```python
from build123d import *

# Parameters (mm, degrees)
SKETCH1_R          = 76.2
EXTRUDE1_DEPTH     = 17.272
SKETCH2_R          = 30.099
CUT_EXTRUDE1_DEPTH = 22.352
SKETCH3_R          = 4.2164
CUT_EXTRUDE3_DEPTH = 22.352
CIRPATTERN1_COUNT  = 8
SKETCH4_R          = 4.2164
CUT_EXTRUDE4_DEPTH = 22.352
CIRPATTERN2_COUNT  = 16


with BuildPart() as part:
    # Sketch1 → Extrude1 (new body)
    with BuildSketch(Plane(origin=(0, 0, 0), x_dir=(1, 0, 0), z_dir=(0, 1, 0))):
        with Locations(Location((0, 0, 0), (0, 0, 270))):
            Circle(SKETCH1_R)
    extrude(amount=EXTRUDE1_DEPTH)

    # Sketch2 → Cut-Extrude1 (cut)
    with BuildSketch(Plane(origin=(0, 0, 0), x_dir=(1, 0, 0), z_dir=(0, 1, 0))):
        with Locations(Location((0, 0, 0), (0, 0, 270))):
            Circle(SKETCH2_R)
    extrude(amount=CUT_EXTRUDE1_DEPTH, mode=Mode.SUBTRACT)

    # Sketch3 → Cut-Extrude3 (cut)
    with BuildSketch(Plane(origin=(0, 0, 0), x_dir=(1, 0, 0), z_dir=(0, 1, 0))):
        with Locations(Location((0, 46.101, 0), (0, 0, 270))):
            Circle(SKETCH3_R)
    cut_extrude3 = extrude(amount=CUT_EXTRUDE3_DEPTH, mode=Mode.SUBTRACT)

    # CirPattern1: Cut-Extrude3 ×8 about axis
    cirpattern1_axis = Axis((0, 0, 0), (0, 1, 0))
    for i in range(1, CIRPATTERN1_COUNT):
        add(cut_extrude3.rotate(cirpattern1_axis, i * 360 / CIRPATTERN1_COUNT), mode=Mode.SUBTRACT)

    # Sketch4 → Cut-Extrude4 (cut)
    with BuildSketch(Plane(origin=(0, 0, 0), x_dir=(1, 0, 0), z_dir=(0, 1, 0))):
        with Locations(Location((0, 65.151, 0), (0, 0, 270))):
            Circle(SKETCH4_R)
    cut_extrude4 = extrude(amount=CUT_EXTRUDE4_DEPTH, mode=Mode.SUBTRACT)

    # CirPattern2: Cut-Extrude4 ×16 about axis
    cirpattern2_axis = Axis((0, 0, 0), (0, 1, 0))
    for i in range(1, CIRPATTERN2_COUNT):
        add(cut_extrude4.rotate(cirpattern2_axis, i * 360 / CIRPATTERN2_COUNT), mode=Mode.SUBTRACT)


solid = part.part
```
Model file for the job. Use its own axes, mm. Give positions to 0.01 mm unless a question says otherwise; leave off trailing zeros. Order: outer loops, then holes, each group sorted by start corner. A loop starts at its lowest first (then second) coordinate and runs counter-clockwise, first axis right, second up.
1) Saw through at C-C, the plane x = 33.5. Write the cut outline in (y, z).
2) Mould opens along Z. For faces 1 (the cylindrical face through (-46.367, 8.515, -60.47)), 2 (the flat face through (1, 0, 33)), 3 (the cylindrical face through (-1.27, 8.52, 61.13)) say: +Z half, -Z half, draft (parallel to the pull), parting line (faces both ways), or undercut.
3) Saw through at B-B, the plane x = 0. Write the cut outline in (y, z).
4) Pin check, flat tips, straight feed: pin 1 (6 mm diameter, centred on x = 37.5, y = 12.5, fed in from -Z); pin 2 (3 mm diameter, centred on y = 13.5, z = 13.5, fed in from -X); pin 3 (13.5 mm diameter, centred on x = 24.93, z = 60.19, fed in from -Y); pin 4 (8 mm diameter, centred on y = 3, z = -39, fed in from +X). Stop position of each tip, or through.
5) Saw through at A-A, the plane z = 0. Write the cut outline in (x, y).
6) Wall check: probe 1 along Z at (x, y) = (22, 14.75); probe 2 along Z at (x, y) = (-3.5, 1.75); probe 3 along X at (y, z) = (4.25, -47.5). Give the ranges that are in metal, low to high.
7) Saw through at D-D, the plane y = 15.5. Count the separate pieces of the cut face and the enclosed holes in it, then the cut area to 3 significant figures.
Computed:
1. outline: (0, -68.44) - (17.27, -68.44) - (17.27, -36.72) - (0, -36.72) - close; (0, -28.48) - (17.27, -28.48) - (17.27, 28.48) - (0, 28.48) - close; (0, 36.72) - (17.27, 36.72) - (17.27, 68.44) - (0, 68.44) - close
2. face 1: parting line
2. face 2: draft
2. face 3: undercut
3. outline: (0, -76.2) - (17.27, -76.2) - (17.27, -69.37) - (0, -69.37) - close; (0, -60.93) - (17.27, -60.93) - (17.27, -50.32) - (0, -50.32) - close; (0, -41.88) - (17.27, -41.88) - (17.27, -30.1) - (0, -30.1) - close; (0, 30.1) - (17.27, 30.1) - (17.27, 41.88) - (0, 41.88) - close; (0, 50.32) - (17.27, 50.32) - (17.27, 60.93) - (0, 60.93) - close; (0, 69.37) - (17.27, 69.37) - (17.27, 76.2) - (0, 76.2) - close
4. pin 1: stops at z = -67.94
4. pin 2: stops at x = -75.25
4. pin 3: stops at y = 0
4. pin 4: stops at x = 67.69
5. outline: (-76.2, 0) - (-69.37, 0) - (-69.37, 17.27) - (-76.2, 17.27) - close; (-60.93, 0) - (-50.32, 0) - (-50.32, 17.27) - (-60.93, 17.27) - close; (-41.88, 0) - (-30.1, 0) - (-30.1, 17.27) - (-41.88, 17.27) - close; (30.1, 0) - (41.88, 0) - (41.88, 17.27) - (30.1, 17.27) - close; (50.32, 0) - (60.93, 0) - (60.93, 17.27) - (50.32, 17.27) - close; (69.37, 0) - (76.2, 0) - (76.2, 17.27) - (69.37, 17.27) - close
6. probe 1: z = -72.96 to -63.22, -57.16 to -20.54, 20.54 to 57.16, 63.22 to 72.96
6. probe 2: z = -76.12 to -67.5, -62.8 to -48.45, -43.75 to -29.89, 29.89 to 43.75, 48.45 to 62.8, 67.5 to 76.12
6. probe 3: x = -59.58 to -50.03, -42.1 to -3.98, 3.98 to 42.1, 50.03 to 59.58
7. separate pieces: 1
7. enclosed holes: 25
7. area: 14,100 mm2
